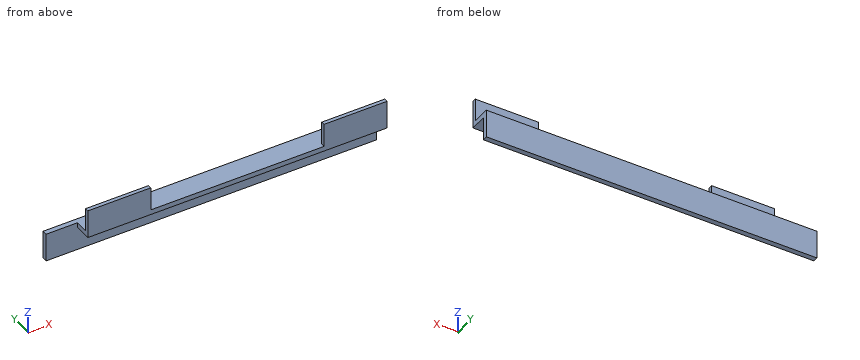
```python
from build123d import *

# Parameters (mm, degrees)
SKETCH1_W           = 2
SKETCH1_H           = 1.5
SKETCH1_W_2         = 9.525
BOSS_EXTRUDE1_DEPTH = 120.65
SKETCH2_W           = 69.85
SKETCH2_H           = 9.525
CUT_EXTRUDE1_DEPTH  = 9.825996
SKETCH3_W           = 11.525
SKETCH3_H           = 2
BOSS_EXTRUDE3_DEPTH = 12.7


with BuildPart() as part:
    # Sketch1 → Boss-Extrude1 (new body)
    with BuildSketch(Plane(origin=(0, 0, 0), x_dir=(0, 0, -1), z_dir=(1, 0, 0))):
        Polygon((-2, 8.825996), (-2, 1.5), (0, 1.5), (0, 6.825996), (9.525, 6.825996), (9.525, 8.825996), align=None)
        with Locations((-1, 0.75)):
            Rectangle(SKETCH1_W, SKETCH1_H)
        with Locations((-6.7625, 0.75)):
            Rectangle(SKETCH1_W_2, SKETCH1_H)
    extrude(amount=BOSS_EXTRUDE1_DEPTH)

    # Sketch2 → Cut-Extrude1 (cut, through all)
    with BuildSketch(Plane.XZ):
        with Locations((60.325, 6.7625)):
            Rectangle(SKETCH2_W, SKETCH2_H)
    extrude(amount=-CUT_EXTRUDE1_DEPTH, mode=Mode.SUBTRACT)

    # Sketch3 → Boss-Extrude3 (add)
    with BuildSketch(Plane.ZY):
        with Locations((-3.7625, 7.825996)):
            Rectangle(SKETCH3_W, SKETCH3_H)
    extrude(amount=BOSS_EXTRUDE3_DEPTH)


solid = part.part
```
The listing builds one solid part. Answer for the finished solid, in the listing's coordinates (mm). Coordinates: 2 decimals unless noted, no trailing zeros. Write each loop counter-clockwise with the first axis right and the second up, starting at its lowest first coordinate (ties: lowest second). Pieces come first, ordered by that corner, then holes. Notation, with made-up numbers: (28.25, -17.5) - (36.25, -17.5) arc R11 ccw to (36.25, -2.5) - close; hole circle Ø11 at (87, 79.5). An arc over 180 degrees is marked (long way). One line per item, written item: value.
1) Find section D-D (z = -6.5). Give the vertices of the cut face in (x, y), and give its area (3 significant figures).
Geometry check:
outline: (-12.7, 6.83) - (120.65, 6.83) - (120.65, 8.83) - (-12.7, 8.83) - close
area: 267 mm2
2) Find section B-B (x = 105). Give the vertices of the cut face in (y, z) (3 decimals), and give its area (3 significant figures).
Geometry check:
outline: (0, 0) - (6.826, 0) - (6.826, -9.525) - (8.826, -9.525) - (8.826, 2) - (1.5, 2) - (1.5, 11.525) - (0, 11.525) - close
area: 51.0 mm2
3) Each of these flat-tipped pins is pushed along its axis until it touches: pin 1 Ø3.5 at (x, z) = (46, -5) entering from -Y; pin 2 Ø5 at (x, z) = (18, 8.5) entering from +Y; pin 3 Ø4 at (y, z) = (5.5, 5.5) entering from -X; pin 4 Ø2 at (x, y) = (52.5, 4) entering from -Z. Where does it stop, or does it pass through?
Geometry check:
pin 1: stops at y = 6.83
pin 2: stops at y = 1.5
pin 3: passes through
pin 4: stops at z = 0
4) Consider line 1 along X through (y, z) = (0.5, 8.25); line 2 along Y through (x, z) = (103, -8.5); line 3 along Z through (x, y) = (24, 7.25) (3 decimals). Determine where each line is inside the solid, lowest interval first. Write a range as from..to.
Geometry check:
line 1: x = 0..25.4, 95.25..120.65
line 2: y = 6.83..8.83
line 3: z = -9.525..2
5) Find section C-C (y = 4). Give the vertices of the cut face in (x, z), and give its area (3 significant figures).
Geometry check:
outline: (0, 0) - (120.65, 0) - (120.65, 2) - (0, 2) - close
area: 241 mm2
6) Find section A-A (z = 8.5). Give the vertices of the cut face in (x, y), and give its area (3 significant figures).
Geometry check:
outline: (0, 0) - (25.4, 0) - (25.4, 1.5) - (0, 1.5) - close; (95.25, 0) - (120.65, 0) - (120.65, 1.5) - (95.25, 1.5) - close
area: 76.2 mm2
